Source: three-view drawing plus pictorial views. Frame: mm from the lowest corner of the part. Round coordinates to 2 decimals unless told otherwise and drop trailing zeros. Order: outer loops, then holes, each group sorted by start corner. A loop starts at its lowest first (then second) coordinate and runs counter-clockwise, first axis right, second up. Notation, with made-up numbers: M 10.5,-23 L 42.5,-23 A31 cw 42.5,9 Z; hole C -3.5,29 d3. An arc over 180 degrees is marked long. Return JSON: item names as keys, results as strings. Group by question number.
Q1. Cut plane C-C on y = 15.5. Output: boundary loops of the cut face in (x, z) (1 decimal), and give its area (3 significant figures).
Q2. Contact query for flat-ended pins moving along their axis: pin 1 (8 mm diameter, centred on x = 87.5, y = 11.5, fed in from +Z) (3 decimals); pin 2 (1.6 mm diameter, centred on x = 1.5, z = 2, fed in from -Y) (3 decimals); pin 3 (1.6 mm diameter, centred on x = 119.5, z = 1, fed in from +Y) (3 decimals); pin 4 (1.6 mm diameter, centred on y = 13.5, z = 2, fed in from -X) (3 decimals). Output: stop coordinate, or through.
Q3. Ray query, probe 1 along Y at (x, z) = (63, 2.2); probe 2 along X at (y, z) = (16.75, 1.4) (1 decimal); probe 3 along X at (y, z) = (7.25, 2.6). Return the intervals inside material, ascending.
Q4. Cut plane A-A on x = 62. Output: boundary loops of the cut face in (y, z) (1 decimal).
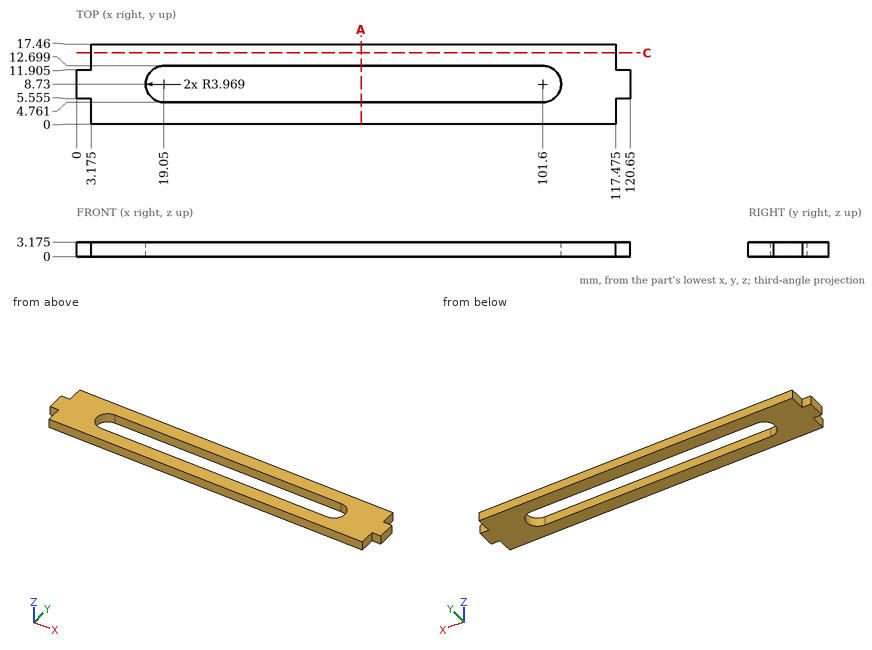
Result sheet:
{
 "1": {"outline": "M 3.2,0 L 117.5,0 L 117.5,3.2 L 3.2,3.2 Z", "area": "363 mm²"},
 "2": {"pin 1": "stops at z = 3.175", "pin 2": "stops at y = 5.555", "pin 3": "stops at y = 11.905", "pin 4": "stops at x = 3.175"},
 "3": {"probe 1": "y = 0 to 4.76, 12.7 to 17.46", "probe 2": "x = 3.2 to 117.5", "probe 3": "x = 0 to 15.37, 105.28 to 120.65"},
 "4": {"outline": "M 0,0 L 4.8,0 L 4.8,3.2 L 0,3.2 Z; M 12.7,0 L 17.5,0 L 17.5,3.2 L 12.7,3.2 Z"}
}
